Could you check a few things on this model? Use its own coordinates, in mm. Face numbers are marked on the shaded views. A direction names the side the tool comes from. Round coordinates to 2 decimals unless told otherwise and drop trailing zeros. Loops run counter-clockwise (first coordinate to the right, second up) from the corner with the lowest first, then second, coordinate; pieces in that order, holes last. Notation, with made-up numbers: (79.5, 50.5) -> (120.5, 50.5) arc R22 cw to (120.5, 75.5) -> close; hole circle Ø10 at (-17.75, 15). An arc over 180 degrees is marked (long way). Use CSV: the item, a comma, the result in double quotes. Start each with the question number.
```python
from build123d import *

# Parameters (mm, degrees)
CROQUIS1_W              = 40
CROQUIS1_H              = 20
SALIENTE_EXTRUIR1_DEPTH = 29.4
SALIENTE_EXTRUIR2_DEPTH = 2.1
CROQUIS3_R              = 2
CORTAR_EXTRUIR1_DEPTH   = 2.1
SALIENTE_EXTRUIR3_DEPTH = 6
CROQUIS5_R              = 10.001656383
SALIENTE_EXTRUIR4_DEPTH = 2
CROQUIS6_R              = 6.45
SALIENTE_EXTRUIR5_DEPTH = 2
CROQUIS7_R              = 2.9
SALIENTE_EXTRUIR6_DEPTH = 4


with BuildPart() as part:
    # Croquis1 → Saliente-Extruir1 (new body)
    with BuildSketch(Plane(origin=(0, 0, 0), x_dir=(1, 0, 0), z_dir=(0, 1, 0))):
        with Locations((20, -10)):
            Rectangle(CROQUIS1_W, CROQUIS1_H)
    extrude(amount=SALIENTE_EXTRUIR1_DEPTH)

    # Croquis2 → Saliente-Extruir2 (add)
    with BuildSketch(Plane(origin=(0, 29.4, 0), x_dir=(1, 0, 0), z_dir=(0, 1, 0))):
        Polygon((20, 0), (-7.2, 0), (-7.2, -20.003312767), (47.2, -20.003312767), (47.2, 0), align=None)
    extrude(amount=SALIENTE_EXTRUIR2_DEPTH)

    # Croquis3 → Cortar-Extruir1 (cut)
    with BuildSketch(Plane(origin=(0, 31.5, 0), x_dir=(1, 0, 0), z_dir=(0, 1, 0))):
        with Locations(Location((-4.095776159, -5.000828192, 0), (0, 0, 270))):
            Circle(CROQUIS3_R)
        with Locations(Location((-4.095776159, -15.002484575, 0), (0, 0, 270))):
            Circle(CROQUIS3_R)
        with Locations(Location((44.010481376, -5.000828192, 0), (0, 0, 270))):
            Circle(CROQUIS3_R)
        with Locations(Location((44.010481376, -15.002484575, 0), (0, 0, 270))):
            Circle(CROQUIS3_R)
    extrude(amount=-CORTAR_EXTRUIR1_DEPTH, mode=Mode.SUBTRACT)

    # Croquis4 → Saliente-Extruir3 (add)
    with BuildSketch(Plane(origin=(0, 31.5, 0), x_dir=(1, 0, 0), z_dir=(0, 1, 0))):
        Polygon((0, 0), (0, -20.003312767), (40.001626581, -20.003312767), (40, 0), align=None)
    extrude(amount=SALIENTE_EXTRUIR3_DEPTH)

    # Croquis5 → Saliente-Extruir4 (add)
    with BuildSketch(Plane(origin=(0, 37.5, 0), x_dir=(1, 0, 0), z_dir=(0, 1, 0))):
        with Locations(Location((29.510368289, -10.001656383, 0), (0, 0, 270))):
            Circle(CROQUIS5_R)
    extrude(amount=SALIENTE_EXTRUIR4_DEPTH)

    # Croquis6 → Saliente-Extruir5 (add)
    with BuildSketch(Plane(origin=(0, 39.5, 0), x_dir=(1, 0, 0), z_dir=(0, 1, 0))):
        with Locations(Location((29.510368289, -10.001656383, 0), (0, 0, 270))):
            Circle(CROQUIS6_R)
    extrude(amount=SALIENTE_EXTRUIR5_DEPTH)

    # Croquis7 → Saliente-Extruir6 (add)
    with BuildSketch(Plane(origin=(0, 41.5, 0), x_dir=(1, 0, 0), z_dir=(0, 1, 0))):
        with Locations(Location((29.510368289, -10.001656383, 0), (0, 0, 270))):
            Circle(CROQUIS7_R)
    extrude(amount=SALIENTE_EXTRUIR6_DEPTH)


solid = part.part
```
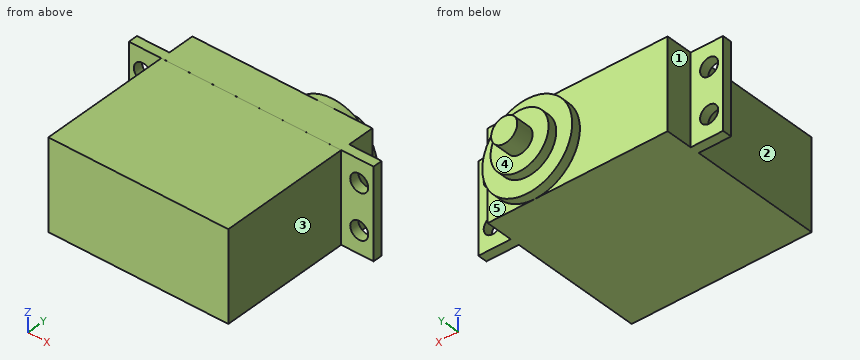
1. For the marked faces 1, 2, 3, 4 and 5, which set-ups out of +Z, -Z, +X, -X, +Y, -Y let a thin tool reach every point of the face, with its end or its side?
2. Suppose I cut it at D-D (z = 10.5). List the corners of the cut face in (x, y) for me.
3. If I drill on L1, parallel to X at y = 10, z = 1; L2, parallel to Z at x = 15, y = 7; L3, parallel to Y at x = 17, z = 17.5, over which ranges is the centre line in solid material (lowest first)?
4. Suppose I cut it at C-C (y = 36.5). List the corners of the cut face in (x, z) for me, then the cut area to 3 significant figures.
5. Will these pins go through, and if not, where does the flat tip stop? pin 1 (11.5 mm diameter, centred on x = 35, z = 6, fed in from +Y); pin 2 (4 mm diameter, centred on y = 6.5, z = 17.5, fed in from -X); pin 3 (5 mm diameter, centred on x = 17.5, y = 10, fed in from +Z); pin 4 (1.5 mm diameter, centred on y = 24, z = 2.5, fed in from +X).
6. Suppose I cut it at A-A (z = 5.5). List the corners of the cut face in (x, y) for me.
Geometry check:
1,face 1,"+Z, -Z, -X, +Y"
1,face 2,"+Z, -Z, -X, -Y"
1,face 3,"+Z, -Z, +X, -Y"
1,face 4,"+Y"
1,face 5,"+X, +Y"
2,outline,"(-7.2, 29.4) -> (0, 29.4) -> (0, 0) -> (40, 0) -> (40, 29.4) -> (47.2, 29.4) -> (47.2, 31.5) -> (40, 31.5) -> (40, 37.5) -> (39.5, 37.5) -> (39.5, 39.5) -> (35.94, 39.5) -> (35.94, 41.5) -> (32.37, 41.5) -> (32.37, 45.5) -> (26.65, 45.5) -> (26.65, 41.5) -> (23.08, 41.5) -> (23.08, 39.5) -> (19.52, 39.5) -> (19.52, 37.5) -> (0, 37.5) -> (0, 31.5) -> (-7.2, 31.5) -> close"
3,L1,"x = 0 to 40"
3,L2,"z = 0 to 20"
3,L3,"y = 0 to 37.5"
4,outline,"(0, 0) -> (40, 0) -> (40, 20) -> (0, 20) -> close"
4,area,"800 mm²"
5,pin 1,"stops at y = 45.5"
5,pin 2,"stops at x = 0"
5,pin 3,"stops at z = 20"
5,pin 4,"stops at x = 40"
6,outline,"(-7.2, 29.4) -> (-6.03, 29.4) -> (-6.03, 31.5) -> (-7.2, 31.5) -> close; (-2.16, 29.4) -> (0, 29.4) -> (0, 0) -> (40, 0) -> (40, 29.4) -> (42.07, 29.4) -> (42.07, 31.5) -> (40, 31.5) -> (40, 37.5) -> (38.44, 37.5) -> (38.44, 39.5) -> (34.13, 39.5) -> (34.13, 41.5) -> (24.89, 41.5) -> (24.89, 39.5) -> (20.58, 39.5) -> (20.58, 37.5) -> (0, 37.5) -> (0, 31.5) -> (-2.16, 31.5) -> close; (45.95, 29.4) -> (47.2, 29.4) -> (47.2, 31.5) -> (45.95, 31.5) -> close"
